Check sheet for the modelled part. Datum: model origin and axes. Units: mm. Face numbers are marked on the shaded views. A direction names the side the tool comes from. Coordinates: 2 decimals unless noted, no trailing zeros. Write each loop counter-clockwise with the first axis right and the second up, starting at its lowest first coordinate (ties: lowest second). Pieces come first, ordered by that corner, then holes. Notation, with made-up numbers: (55, -35) -> (70, -35) arc R5 cw to (70, -26) -> close; hole circle Ø10 at (15.5, 16.25). An arc over 180 degrees is marked (long way). One line per item, written item: value. Start each with the question number.
1) Sectioned sample at C-C on z = 0.75. Enter the section's corners in (x, y) (3 decimals), plus the area to 3 significant figures.
2) Set-up check for the marked faces 1, 2, 3, 4 and 5: record each of +Z, -Z, +X, -X, +Y, -Y from which the full face is reachable in a straight line by a thin tool's end or side.
3) Sectioned sample at A-A on x = -1.75. Enter the section's corners in (y, z), plus the area to 3 significant figures.
4) Draft check along X on the marked faces 6, 7 and 8. Enter one of: +X half, -X half, draft (parallel to the pull), parting line (faces both ways), or undercut.
5) Sectioned sample at D-D on x = -1. Enter the section's corners in (y, z).
6) Gauge pin test, flat ends, axial feed: P1, Ø1.7, axis at x = 0.5, z = 0, coming from the -Y side; P2, Ø0.7, axis at x = 1.5, y = 4.5, coming from the +Z side. Record the tip position at first contact, or that the pin passes through.
7) Scan lines: line 1 along X through (y, z) = (7.5, 1) (3 decimals); line 2 along Z through (x, y) = (2.25, 5.25); line 3 along Z through (x, y) = (-1.25, 4.5). Record each from-to range of solid material in increasing order. Write a range as [from, to].
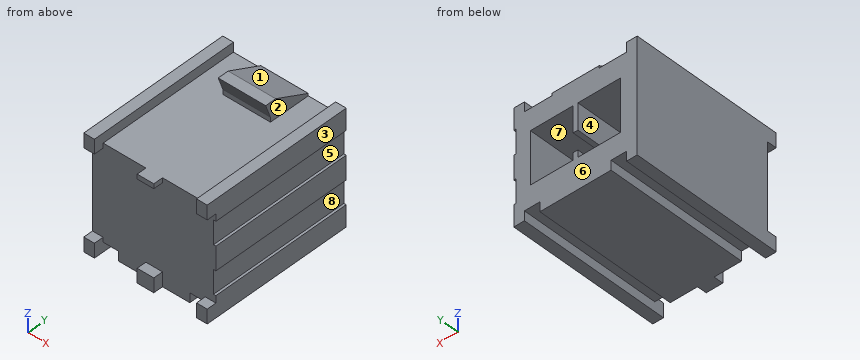
Autodesk Inventor part; units mm, degrees
ref_plane "header_to_dummy_XY" through (0, 0, 0) normal (0, -1, 0) x (1, 0, 0)
ref_plane "header_to_dummy_YZ" through (0, 0, 0) normal (1, 0, 0) x (0, 0, 1)
ref_plane "header_to_dummy_ZX" through (0, 0, 0) normal (0, 0, 1) x (0, -1, 0)
sketch "Sketch_1" plane through (0, 0, 0) normal (1, 0, 0) x (0, 1, 0)
  line L0 (8.128, 3.048) -> (0, 3.048)
  line L1 (0, 3.048) -> (0, 2.286)
  line L2 (0, 2.286) -> (0.508, 2.286)
  line L3 (0.508, 2.286) -> (0.508, -2.286)
  line L4 (0.508, -2.286) -> (0, -2.286)
  line L5 (0, -2.286) -> (0, -3.048)
  line L6 (0, -3.048) -> (8.128, -3.048)
  line L7 (8.128, -3.048) -> (8.128, 3.048)
extrude "Extrusion1" add sketch "Sketch_1" along normal mid plane 6.604
sketch "Sketch_4" plane through (0, 0, 0) normal (0, 0, 1) x (1, 0, 0)
  line L0 (-2.7305, 0.508) -> (-2.7305, -0.508)
  line L1 (-2.7305, -0.508) -> (-0.4445, -0.508)
  line L2 (-0.4445, -0.508) -> (-0.4445, 0.508)
  line L3 (-0.4445, 0.508) -> (-2.7305, 0.508)
extrude "Extrusion2" cut sketch "Sketch_4" along normal mid plane 6.096
sketch "Sketch_5" plane through (0, 0, 0) normal (0, 0, 1) x (1, 0, 0)
  line L0 (0.4445, 0.508) -> (0.4445, -0.508)
  line L1 (0.4445, -0.508) -> (2.7305, -0.508)
  line L2 (2.7305, -0.508) -> (2.7305, 0.508)
  line L3 (2.7305, 0.508) -> (0.4445, 0.508)
extrude "Extrusion3" cut sketch "Sketch_5" along normal mid plane 6.096
sketch "Sketch_9" plane through (0, 8.128, 0) normal (0, 1, 0) x (1, 0, 0)
  line L0 (-2.4117, 1.3945) -> (-2.4117, -1.397)
  line L1 (-2.4117, -1.397) -> (-0.1283, -1.397)
  line L2 (-0.1283, -1.397) -> (-0.1283, 1.3945)
  line L3 (-0.1283, 1.3945) -> (-2.4117, 1.3945)
extrude "Extrusion4" cut sketch "Sketch_9" against normal blind 5.842
pattern_linear "Rectangular Pattern1" count 2 spacing 2.54 along (1, 0, -0.001) of "Extrusion4"
sketch "Sketch_21" plane through (0, 0, 0) normal (0, 1, 0) x (-1, 0, 0)
  line L0 (3.81, -3.81) -> (3.81, 3.556)
  line L1 (3.81, 3.556) -> (-3.81, 3.556)
  line L2 (-3.81, 3.556) -> (-3.81, -3.81)
  line L3 (-3.81, -3.81) -> (3.81, -3.81)
  line L4 (3.302, -3.048) -> (3.302, 3.048)
  line L5 (3.302, 3.048) -> (2.7305, 3.048)
  line L6 (2.7305, 3.048) -> (2.7305, 2.54)
  line L7 (2.7305, 2.54) -> (-2.7305, 2.54)
  line L8 (-2.7305, 2.54) -> (-2.7305, 3.048)
  line L9 (-2.7305, 3.048) -> (-3.302, 3.048)
  line L10 (-3.302, 3.048) -> (-3.302, -3.048)
  line L11 (-3.302, -3.048) -> (-2.7305, -3.048)
  line L12 (-2.7305, -3.048) -> (-2.7305, -2.54)
  line L13 (-2.7305, -2.54) -> (-1.905, -2.54)
  line L14 (-1.905, -2.54) -> (-1.905, -3.048)
  line L15 (-1.905, -3.048) -> (1.905, -3.048)
  line L16 (1.905, -3.048) -> (1.905, -2.54)
  line L17 (1.905, -2.54) -> (2.7305, -2.54)
  line L18 (2.7305, -2.54) -> (2.7305, -3.048)
  line L19 (2.7305, -3.048) -> (3.302, -3.048)
extrude "Extrusion5" cut sketch "Sketch_21" along normal blind 8.128
sketch "Sketch_25" plane through (0, 0, 0) normal (1, 0, 0) x (0, 1, 0)
  line L0 (6.223, 3.556) -> (5.6388, 3.556)
  line L1 (5.6388, 3.556) -> (5.9182, 2.794)
  line L2 (5.9182, 2.794) -> (5.9182, 2.54)
  line L3 (5.9182, 2.54) -> (8.128, 2.54)
  line L4 (8.128, 2.54) -> (8.128, 2.667)
  line L5 (8.128, 2.667) -> (6.223, 3.556)
extrude "Extrusion6" add sketch "Sketch_25" along normal mid plane 2.54
sketch "Sketch_26" plane through (0, 8.128, 0) normal (0, 1, 0) x (1, 0, 0)
  line L0 (-0.508, 1.016) -> (-0.508, 0)
  line L1 (-0.508, 0) -> (0.508, 0)
  line L2 (0.508, 0) -> (0.508, 1.016)
  line L3 (0.508, 1.016) -> (-0.508, 1.016)
extrude "Extrusion7" cut sketch "Sketch_26" against normal blind 5.842
sketch "Sketch_38" plane through (0, 0, 0) normal (0, 1, 0) x (-1, 0, 0)
  line L0 (-3.175, 0.635) -> (-3.175, 1.905)
  line L1 (-3.175, 1.905) -> (-3.556, 1.905)
  line L2 (-3.556, 1.905) -> (-3.556, -1.905)
  line L3 (-3.556, -1.905) -> (-3.175, -1.905)
  line L4 (-3.175, -1.905) -> (-3.175, -0.635)
  line L5 (-3.175, -0.635) -> (-3.429, -0.635)
  line L6 (-3.429, -0.635) -> (-3.429, 0.635)
  line L7 (-3.429, 0.635) -> (-3.175, 0.635)
extrude "Extrusion8" cut sketch "Sketch_38" along normal blind 8.128
ref_plane "header_to_dummy_XY" through (0, 0, 0) normal (0, -1, 0) x (1, 0, 0)
ref_plane "header_to_dummy_YZ" through (0, 0, 0) normal (1, 0, 0) x (0, 0, 1)
ref_plane "header_to_dummy_ZX" through (0, 0, 0) normal (0, 0, 1) x (0, -1, 0)
ref_plane "header_to_pad_XY" through (0, 8.128, 0) normal (0, 1, 0) x (1, 0, 0)
ref_plane "header_to_pad_YZ" through (0, 8.128, 0) normal (1, 0, 0) x (0, 0, -1)
ref_plane "header_to_pad_ZX" through (0, 8.128, 0) normal (0, 0, -1) x (0, 1, 0)
properties part number "IPL1-102-01-S-K_header"
Answers:
1. outline: (-3.302, 0.508) -> (3.175, 0.508) -> (3.175, 8.128) -> (2.412, 8.128) -> (2.412, 2.286) -> (0.128, 2.286) -> (0.128, 8.128) -> (-0.128, 8.128) -> (-0.128, 2.286) -> (-2.412, 2.286) -> (-2.412, 8.128) -> (-3.302, 8.128) -> close
1. area: 22.7 mm2
2. face 1: +Z, +Y
2. face 2: +Z, +Y, -Y
2. face 3: +Z, -Z, +X, +Y, -Y
2. face 4: +Y
2. face 5: +X, +Y, -Y
3. outline: (0.51, -3.05) -> (8.13, -3.05) -> (8.13, -1.39) -> (2.29, -1.39) -> (2.29, 1.4) -> (8.13, 1.4) -> (8.13, 2.54) -> (0.51, 2.54) -> close
3. area: 26.3 mm2
4. face 6: draft
4. face 7: undercut
4. face 8: +X half
5. outline: (0.51, -3.05) -> (8.13, -3.05) -> (8.13, -1.39) -> (2.29, -1.39) -> (2.29, 1.4) -> (8.13, 1.4) -> (8.13, 2.67) -> (6.22, 3.56) -> (5.64, 3.56) -> (5.92, 2.79) -> (5.92, 2.54) -> (0.51, 2.54) -> close
6. P1: stops at y = 0.51
6. P2: stops at z = 2.54
7. line 1: x = [-3.302, -2.412], [-0.128, 0.128], [2.412, 3.175]
7. line 2: z = [-2.54, -1.4], [1.39, 2.54]
7. line 3: z = [-3.05, -1.39], [1.4, 2.54]
